```python
from build123d import *

# Parameters (mm, degrees)
BOSS_EXTRUDE1_DEPTH = 11.5
SKETCH2_R           = 3.15
BOSS_EXTRUDE2_DEPTH = 7.8
SKETCH3_R           = 1.8
BOSS_EXTRUDE3_DEPTH = 1


with BuildPart() as part:
    # Sketch1 → Boss-Extrude1 (new body)
    with BuildSketch(Plane.XY):
        with BuildLine():
            Line((-26, 21), (-26, -21))
            ThreePointArc((-26, -21), (-20.142135624, -35.142135624), (-6, -41))
            Line((-6, -41), (6, -41))
            ThreePointArc((6, -41), (20.142135624, -35.142135624), (26, -21))
            Line((26, -21), (26, 21))
            ThreePointArc((26, 21), (20.142135624, 35.142135624), (6, 41))
            Line((6, 41), (-6, 41))
            ThreePointArc((-6, 41), (-20.142135624, 35.142135624), (-26, 21))
        make_face()
    extrude(amount=BOSS_EXTRUDE1_DEPTH)

    # Sketch2 → Boss-Extrude2 (add)
    with BuildSketch(Plane(origin=(0, 41, 0), x_dir=(1, 0, 0), z_dir=(0, 1, 0))):
        with Locations(Location((0, -7, 0), (0, 0, 90))):
            Circle(SKETCH2_R)
    boss_extrude2 = extrude(amount=BOSS_EXTRUDE2_DEPTH)

    # Sketch3 → Boss-Extrude3 (add, symmetric)
    with BuildSketch(Plane(origin=(0, 41, 0), x_dir=(1, 0, 0), z_dir=(0, 1, 0))):
        with Locations(Location((-6, -7, 0), (0, 0, 270))):
            Circle(SKETCH3_R)
        with Locations(Location((6, -7, 0), (0, 0, 270))):
            Circle(SKETCH3_R)
    boss_extrude3 = extrude(amount=BOSS_EXTRUDE3_DEPTH, both=True)

    # Mirror1: Boss-Extrude2, Boss-Extrude3 across plane
    add(boss_extrude2.mirror(Plane.ZX))
    add(boss_extrude3.mirror(Plane.ZX))


solid = part.part
```
Could you check a few things on this model? Use its own coordinates, in mm. A direction names the side the tool comes from. Coordinates: 2 decimals unless noted, no trailing zeros. Loops run counter-clockwise (first coordinate to the right, second up) from the corner with the lowest first, then second, coordinate; pieces in that order, holes last.
1) Imagine slicing it at B-B (x = 0). List the corners of the cut face in (y, z) for me, and give its area (3 significant figures).
Reported:
outline: (-48.8, 3.85) - (-41, 3.85) - (-41, 0) - (41, 0) - (41, 3.85) - (48.8, 3.85) - (48.8, 10.15) - (41, 10.15) - (41, 11.5) - (-41, 11.5) - (-41, 10.15) - (-48.8, 10.15) - close
area: 1,040 mm2
2) Which directions (+Z, -Z, +X, -X, +Y, -Y) give clear straight access to the entire face, cutting with the end or side of a thin tool? Please do faces 4 (the face through (7.785, 41.467, 6.766)), 5 (the face through (-6, 42, 7)), 6 (the face through (6, -42, 7)).
Reported:
face 4: +Y
face 5: +Z, -Z, -X, +Y
face 6: +Z, -Z, +X, -Y
3) Please list where these lines run through material, in increasing order: line 1 along X through (y, z) = (21.5, 10.5); line 2 along Y through (x, z) = (4, 10.75); line 3 along Y through (x, z) = (-22, 10.75).
Reported:
line 1: x = -25.99 to 25.99
line 2: y = -41 to 41
line 3: y = -33 to 33
4) Thinking about a two-plate mould opening in X: for faces 1 (the face through (26, 0, 6)), 2 (the face through (-7.757, -41.452, 6.61)), 3 (the face through (0, -48.8, 7)), which applies, released by +X, released by -X, zero draft, split by the parting line, or undercut?
Reported:
face 1: released by +X
face 2: undercut
face 3: zero draft
5) Imagine slicing it at D-D (y = 43). List the corners of the cut face in (x, z) for me.
Reported:
outline: circle Ø6.3 at (0, 7)
6) Imagine slicing it at A-A (z = 7). List the corners of the cut face in (x, y) for me, and give its area (3 significant figures).
Reported:
outline: (-26, -21) arc R20 ccw to (-7.8, -40.92) - (-7.8, -42) - (-4.2, -42) - (-4.2, -41) - (-3.15, -41) - (-3.15, -48.8) - (3.15, -48.8) - (3.15, -41) - (4.2, -41) - (4.2, -42) - (7.8, -42) - (7.8, -40.92) arc R20 ccw to (26, -21) - (26, 21) arc R20 ccw to (7.8, 40.92) - (7.8, 42) - (4.2, 42) - (4.2, 41) - (3.15, 41) - (3.15, 48.8) - (-3.15, 48.8) - (-3.15, 41) - (-4.2, 41) - (-4.2, 42) - (-7.8, 42) - (-7.8, 40.92) arc R20 ccw to (-26, 21) - close
area: 4,030 mm2
7) Imagine slicing it at C-C (z = 1.75). List the corners of the cut face in (x, y) for me.
Reported:
outline: (-26, -21) arc R20 ccw to (-6, -41) - (6, -41) arc R20 ccw to (26, -21) - (26, 21) arc R20 ccw to (6, 41) - (-6, 41) arc R20 ccw to (-26, 21) - close
8) Will these pins go through, and if not, where does the flat tip stop? pin 1 Ø2 at (x, y) = (13, 34) entering from -Z; pin 2 Ø1.8 at (x, z) = (7, 7) entering from -Y; pin 3 Ø2 at (x, z) = (-4, 2) entering from -Y; pin 4 Ø1.1 at (x, z) = (7, 7) entering from +Y.
Reported:
pin 1: stops at z = 0
pin 2: stops at y = -42
pin 3: stops at y = -41
pin 4: stops at y = 42
